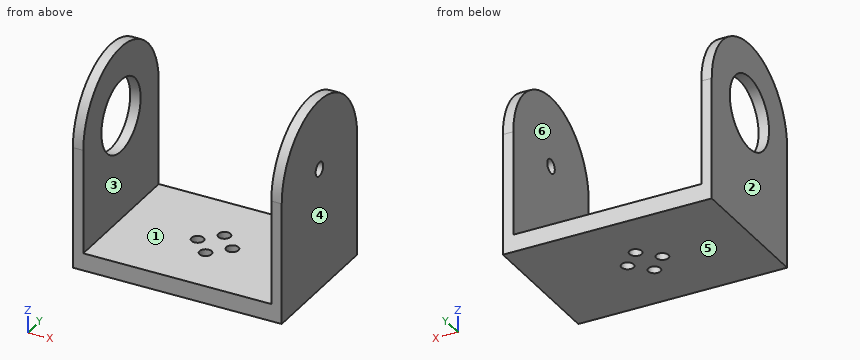
```python
from build123d import *

# Parameters (mm, degrees)
SKETCH1_W               = 60
SKETCH1_H               = 40
BOSS_EXTRUDE1_DEPTH     = 5
SKETCH3_W               = 3
SKETCH3_H               = 40
BOSS_EXTRUDE2_DEPTH     = 30
BOSS_EXTRUDE3_DEPTH     = 3
BOSS_EXTRUDE4_START     = -3
BOSS_EXTRUDE4_DEPTH     = 3
SKETCH8_R               = 1.75
CUT_EXTRUDE1_DEPTH      = 66.76473219
CUT_EXTRUDE2_DEPTH      = 84.815273071
CUT_EXTRUDE2_DEPTH_BACK = 3
SKETCH11_R              = 10.4
SKETCH13_R              = 2
CUT_EXTRUDE3_DEPTH      = 10


with BuildPart() as part:
    # Sketch1 → Boss-Extrude1 (new body)
    with BuildSketch(Plane.XY):
        Rectangle(SKETCH1_W, SKETCH1_H)
    extrude(amount=BOSS_EXTRUDE1_DEPTH)

    # Sketch3 → Boss-Extrude2 (add)
    with BuildSketch(Plane.XY.offset(5)):
        with Locations((-28.5, 0)):
            Rectangle(SKETCH3_W, SKETCH3_H)
        with Locations((28.5, 0)):
            Rectangle(SKETCH3_W, SKETCH3_H)
    extrude(amount=BOSS_EXTRUDE2_DEPTH)

    # Sketch9 → Boss-Extrude3 (add)
    with BuildSketch(Plane(origin=(30, 0, 0), x_dir=(0, 0, -1), z_dir=(1, 0, 0))):
        with BuildLine():
            Line((-35, 20), (-35, -20))
            ThreePointArc((-35, -20), (-55, 0), (-35, 20))
        make_face()
    extrude(amount=-BOSS_EXTRUDE3_DEPTH)

    # Sketch10 → Boss-Extrude4 (add)
    with BuildSketch(Plane.ZY.offset(30).offset(BOSS_EXTRUDE4_START)):
        with BuildLine():
            Line((35, 20), (35, -20))
            ThreePointArc((35, -20), (55, 0), (35, 20))
        make_face()
    extrude(amount=BOSS_EXTRUDE4_DEPTH)

    # Sketch8 → Cut-Extrude1 (cut, through all)
    with BuildSketch(Plane(origin=(0, 0, 0), x_dir=(-1, 0, 0), z_dir=(0, 0, -1))):
        with Locations((-5, 0)):
            Circle(SKETCH8_R)
        with Locations((0, 5)):
            Circle(SKETCH8_R)
        with Locations((0, -5)):
            Circle(SKETCH8_R)
        with Locations((5, 0)):
            Circle(SKETCH8_R)
    extrude(amount=-CUT_EXTRUDE1_DEPTH, mode=Mode.SUBTRACT)

    # Sketch11 → Cut-Extrude2 (cut, two sides: drawn at the far end of the back side and taken through both)
    with BuildSketch(Plane.ZY.offset(30).offset(-CUT_EXTRUDE2_DEPTH_BACK)):
        with Locations(Location((35, 0, 0), (0, 0, 90))):
            Circle(SKETCH11_R)
    extrude(amount=CUT_EXTRUDE2_DEPTH + CUT_EXTRUDE2_DEPTH_BACK, mode=Mode.SUBTRACT)

    # Sketch13 → Cut-Extrude3 (cut)
    with BuildSketch(Plane(origin=(30, 0, 0), x_dir=(0, 0, -1), z_dir=(1, 0, 0))):
        with Locations(Location((-35, 0, 0), (0, 0, 90))):
            Circle(SKETCH13_R)
    extrude(amount=-CUT_EXTRUDE3_DEPTH, mode=Mode.SUBTRACT)


solid = part.part
```
Check sheet for the modelled part. Datum: model origin and axes. Units: mm. Face numbers are marked on the shaded views. A direction names the side the tool comes from. Round coordinates to 2 decimals unless told otherwise and drop trailing zeros. Loops run counter-clockwise (first coordinate to the right, second up) from the corner with the lowest first, then second, coordinate; pieces in that order, holes last. Notation, with made-up numbers: (27, 73.5) - (54, 73.5) arc R22 ccw to (54, 106.5) - close; hole circle Ø8 at (25, -13). An arc over 180 degrees is marked (long way). Write item = value, one per line. Start each with the question number.
Q1. Section check A-A (y = 0). Record the boundary of the cut face in (x, z).
Q2. Section check B-B (x = 0). Record the boundary of the cut face in (y, z), plus the area to 3 significant figures.
Q3. Release check for a two-part mould opening along X. For the marked faces 3, 4, 5 and 6 record: pulls with the +X half, pulls with the -X half, needs draft (parallel to the pull), parting line crosses it, or undercut.
Q4. Section check D-D (y = 5). Record the boundary of the cut face in (x, z), plus the area to 3 significant figures.
Q5. Section check C-C (z = 10). Record the boundary of the cut face in (x, y).
Q6. Access from +Z, -Z, +X, -X, +Y, -Y to the whole of each face (thin tool, end or side, straight path). Record for the marked faces 1 and 2.
Q7. Depth check by flat-ended pin: P1, Ø3, axis at x = -13, y = 4.5, coming from the +Z side; P2, Ø18.5, axis at y = 0, z = 35, coming from the -X side. Enter the tip coordinate at first touch or a pass-through.
Q8. Thickness scan on L1, parallel to Y at x = 0, z = 1; L2, parallel to Z at x = -28, y = 0; L3, parallel to X at y = -13, z = 28.5. Record the ranges inside material, lowest first.
Derived:
q1.outline = (-30, 0) - (-6.75, 0) - (-6.75, 5) - (-27, 5) - (-27, 24.6) - (-30, 24.6) - close; (-30, 45.4) - (-27, 45.4) - (-27, 55) - (-30, 55) - close; (-3.25, 0) - (3.25, 0) - (3.25, 5) - (-3.25, 5) - close; (6.75, 0) - (30, 0) - (30, 33) - (27, 33) - (27, 5) - (6.75, 5) - close; (27, 37) - (30, 37) - (30, 55) - (27, 55) - close
q2.outline = (-20, 0) - (-6.75, 0) - (-6.75, 5) - (-20, 5) - close; (-3.25, 0) - (3.25, 0) - (3.25, 5) - (-3.25, 5) - close; (6.75, 0) - (20, 0) - (20, 5) - (6.75, 5) - close
q2.area = 165 mm^2
q3.face_3 = undercut
q3.face_4 = pulls with the +X half
q3.face_5 = needs draft
q3.face_6 = undercut
q4.outline = (-30, 0) - (-1.75, 0) - (-1.75, 5) - (-27, 5) - (-27, 25.88) - (-30, 25.88) - close; (-30, 44.12) - (-27, 44.12) - (-27, 54.36) - (-30, 54.36) - close; (1.75, 0) - (30, 0) - (30, 54.36) - (27, 54.36) - (27, 5) - (1.75, 5) - close
q4.area = 524 mm^2
q5.outline = (-30, -20) - (-27, -20) - (-27, 20) - (-30, 20) - close; (27, -20) - (30, -20) - (30, 20) - (27, 20) - close
q6.face_1 = +Z, +Y, -Y
q6.face_2 = +Z, -Z, -X, +Y, -Y
q7.P1 = 5
q7.P2 = 27
q8.L1 = -20 to -6.75, -3.25 to 3.25, 6.75 to 20
q8.L2 = 0 to 24.6, 45.4 to 55
q8.L3 = -30 to -27, 27 to 30
